Part print with two shaded views. Sizes in mm from the minimum x, y, z corner. A direction names the side the tool comes from. Coordinates: 2 decimals unless noted, no trailing zeros. Write each loop counter-clockwise with the first axis right and the second up, starting at its lowest first coordinate (ties: lowest second). Pieces come first, ordered by that corner, then holes. Notation, with made-up numbers: (2, -7) - (24, -7) arc R20 cw to (24, -3) - close; hole circle Ø2 at (45.25, 3). An arc over 180 degrees is marked (long way). Answer in a Markdown table with one row per item. Add a question column.
Q1. Band-saw the part on B-B (x = 4.5). List the corners of the cut face in (y, z).
Q2. Two-plate mould, pull along X, no slides. Class the marked faces 3, 4, 5 and 6: +X half, -X half, draft (parallel to the pull), parting line (faces both ways), or undercut.
Q3. Band-saw the part on C-C (z = 5.5). List the corners of the cut face in (x, y).
Q4. 3-axis set-ups, long thin cutter, end or side, ignore diameter. For the marked faces 1 and 2: which of +Z, -Z, +X, -X, +Y, -Y reach the whole face in a straight line?
Q5. Drill centre lines: line 1 along X through (y, z) = (7.25, 7.75); line 2 along Y through (x, z) = (12.5, 16). Where is each one in solid material? Low to high. Write a range as from..to.
Q6. Band-saw the part on A-A (y = 1.5). List the corners of the cut face in (x, z), and give its area (3 significant figures).
Q7. Pin check, flat tips, straight feed: pin 1 (3 mm diameter, centred on x = 14, z = 10.5, fed in from -Y); pin 2 (4 mm diameter, centred on x = 16.5, y = 6, fed in from -Z). Stop position of each tip, or through.
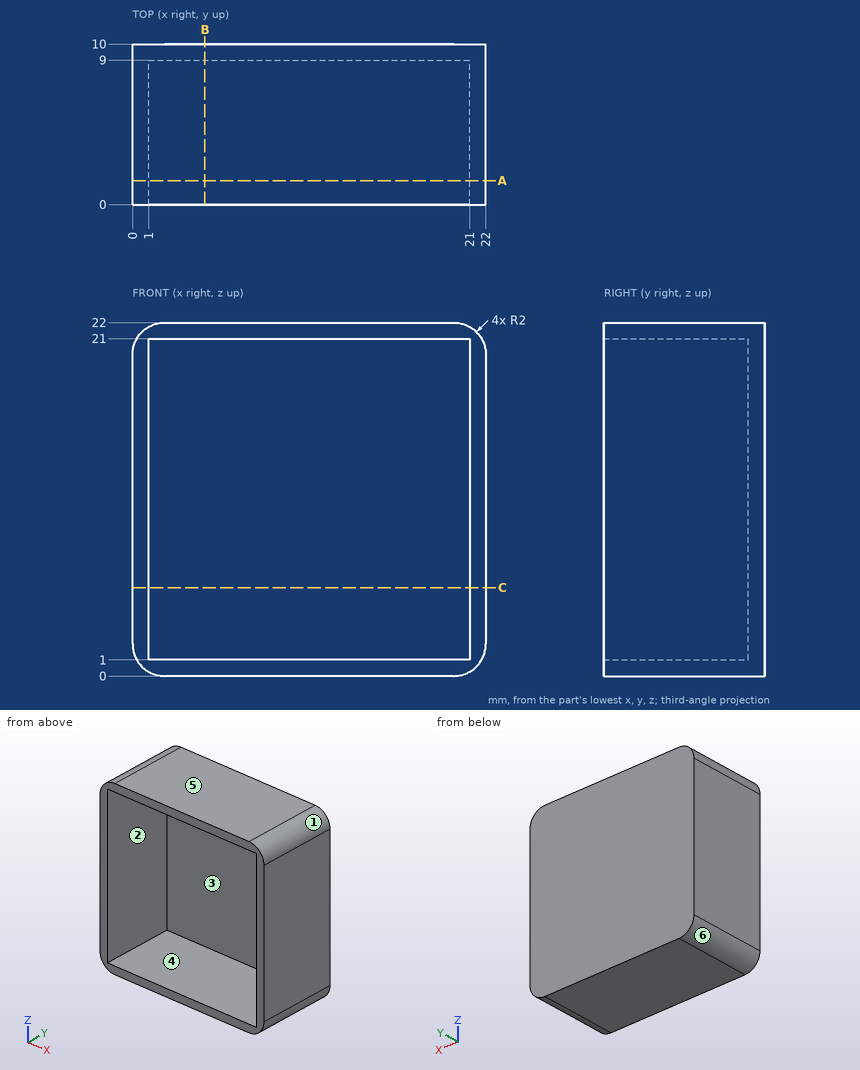
Checked values:
| question | item | result |
|---|---|---|
| 1 | outline | (0, 0) - (10, 0) - (10, 22) - (0, 22) - (0, 21) - (9, 21) - (9, 1) - (0, 1) - close |
| 2 | face 3 | undercut |
| 2 | face 4 | undercut |
| 2 | face 5 | draft |
| 2 | face 6 | -X half |
| 3 | outline | (0, 0) - (1, 0) - (1, 9) - (21, 9) - (21, 0) - (22, 0) - (22, 10) - (0, 10) - close |
| 4 | face 1 | +Z, +X, +Y, -Y |
| 4 | face 2 | -Y |
| 5 | line 1 | x = 0..1, 21..22 |
| 5 | line 2 | y = 9..10 |
| 6 | outline | (0, 2) arc R2 ccw to (2, 0) - (20, 0) arc R2 ccw to (22, 2) - (22, 20) arc R2 ccw to (20, 22) - (2, 22) arc R2 ccw to (0, 20) - close; hole (1, 1) - (21, 1) - (21, 21) - (1, 21) - close |
| 6 | area | 80.6 mm² |
| 7 | pin 1 | stops at y = 9 |
| 7 | pin 2 | stops at z = 0 |
